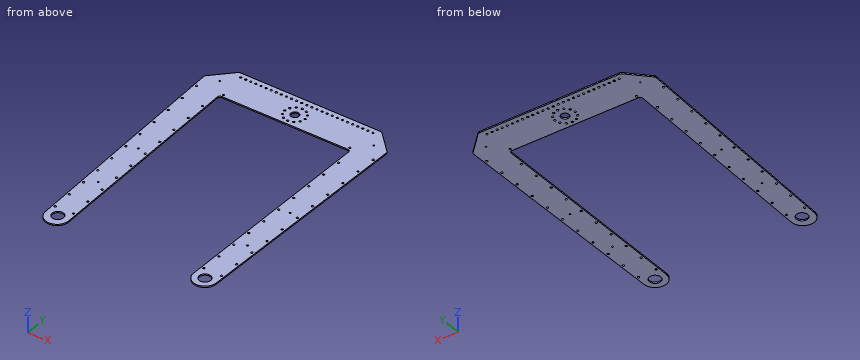
from build123d import *

# Parameters (mm, degrees)
SKETCH1_R           = 14.2875
SKETCH1_R_2         = 2.4892
SKETCH1_R_3         = 1.8288
SKETCH1_R_4         = 10.16
BOSS_EXTRUDE1_DEPTH = 3.175
FILLET1_R           = 6.35


with BuildPart() as part:
    # Sketch1 → Boss-Extrude1 (new body)
    with BuildSketch(Plane.XY):
        with BuildLine():
            Line((431.8, 25.4), (76.2, 25.4))
            Line((76.2, 25.4), (26.059319149, -25.4))
            Line((26.059319149, -25.4), (40.894, -596.9))
            ThreePointArc((40.894, -596.9), (69.687933371, -625.474161286), (98.040645192, -596.462146109))
            Line((98.040645192, -596.462146109), (89.873122894, -63.5))
            Line((89.873122894, -63.5), (418.126877106, -63.5))
            Line((418.126877106, -63.5), (409.959354808, -596.462146109))
            ThreePointArc((409.959354808, -596.462146109), (438.312066629, -625.474161286), (467.106, -596.9))
            Line((467.106, -596.9), (481.940680851, -25.4))
            Line((481.940680851, -25.4), (431.8, 25.4))
        make_face()
        with Locations((69.402383578, -593.962825081)):
            Circle(SKETCH1_R, mode=Mode.SUBTRACT)
        with Locations((46.582379595, -571.328944019)):
            Circle(SKETCH1_R_2, mode=Mode.SUBTRACT)
        with Locations((91.28656025, -570.142707564)):
            Circle(SKETCH1_R_2, mode=Mode.SUBTRACT)
        with Locations((45.264185314, -520.546049618)):
            Circle(SKETCH1_R_2, mode=Mode.SUBTRACT)
        with Locations((43.945991034, -469.763155216)):
            Circle(SKETCH1_R_2, mode=Mode.SUBTRACT)
        with Locations((90.508153333, -519.348671668)):
            Circle(SKETCH1_R_2, mode=Mode.SUBTRACT)
        with Locations((89.729746417, -468.554635771)):
            Circle(SKETCH1_R_2, mode=Mode.SUBTRACT)
        with Locations((67.240460084, -451.479225721)):
            Circle(SKETCH1_R_3, mode=Mode.SUBTRACT)
        with Locations((42.627796754, -418.980260814)):
            Circle(SKETCH1_R_2, mode=Mode.SUBTRACT)
        with Locations((88.9513395, -417.760599874)):
            Circle(SKETCH1_R_2, mode=Mode.SUBTRACT)
        with Locations((41.309602474, -368.197366412)):
            Circle(SKETCH1_R_2, mode=Mode.SUBTRACT)
        with Locations((39.991408193, -317.41447201)):
            Circle(SKETCH1_R_2, mode=Mode.SUBTRACT)
        with Locations((65.373280571, -308.991459085)):
            Circle(SKETCH1_R_3, mode=Mode.SUBTRACT)
        with Locations((88.172932583, -366.966563978)):
            Circle(SKETCH1_R_2, mode=Mode.SUBTRACT)
        with Locations((87.394525667, -316.172528081)):
            Circle(SKETCH1_R_2, mode=Mode.SUBTRACT)
        with Locations((416.71343975, -570.142707564)):
            Circle(SKETCH1_R_2, mode=Mode.SUBTRACT)
        with Locations((438.531, -596.9)):
            Circle(SKETCH1_R, mode=Mode.SUBTRACT)
        with Locations((461.417620405, -571.328944019)):
            Circle(SKETCH1_R_2, mode=Mode.SUBTRACT)
        with Locations((417.491846667, -519.348671668)):
            Circle(SKETCH1_R_2, mode=Mode.SUBTRACT)
        with Locations((418.270253583, -468.554635771)):
            Circle(SKETCH1_R_2, mode=Mode.SUBTRACT)
        with Locations((462.735814686, -520.546049618)):
            Circle(SKETCH1_R_2, mode=Mode.SUBTRACT)
        with Locations((464.054008966, -469.763155216)):
            Circle(SKETCH1_R_2, mode=Mode.SUBTRACT)
        with Locations((419.0486605, -417.760599874)):
            Circle(SKETCH1_R_2, mode=Mode.SUBTRACT)
        with Locations((442.219071981, -454.447733872)):
            Circle(SKETCH1_R_3, mode=Mode.SUBTRACT)
        with Locations((465.372203246, -418.980260814)):
            Circle(SKETCH1_R_2, mode=Mode.SUBTRACT)
        with Locations((419.827067417, -366.966563978)):
            Circle(SKETCH1_R_2, mode=Mode.SUBTRACT)
        with Locations((420.605474333, -316.172528081)):
            Circle(SKETCH1_R_2, mode=Mode.SUBTRACT)
        with Locations((466.690397526, -368.197366412)):
            Circle(SKETCH1_R_2, mode=Mode.SUBTRACT)
        with Locations((445.916762629, -311.995717095)):
            Circle(SKETCH1_R_3, mode=Mode.SUBTRACT)
        with Locations((468.008591807, -317.41447201)):
            Circle(SKETCH1_R_2, mode=Mode.SUBTRACT)
        with Locations((38.673213913, -266.631577608)):
            Circle(SKETCH1_R_2, mode=Mode.SUBTRACT)
        with Locations((86.61611875, -265.378492184)):
            Circle(SKETCH1_R_2, mode=Mode.SUBTRACT)
        with Locations((37.355019633, -215.848683206)):
            Circle(SKETCH1_R_2, mode=Mode.SUBTRACT)
        with Locations((36.036825353, -165.065788804)):
            Circle(SKETCH1_R_2, mode=Mode.SUBTRACT)
        with Locations((85.837711834, -214.584456288)):
            Circle(SKETCH1_R_2, mode=Mode.SUBTRACT)
        with Locations((85.059304917, -163.790420391)):
            Circle(SKETCH1_R_2, mode=Mode.SUBTRACT)
        with Locations((34.718631073, -114.282894402)):
            Circle(SKETCH1_R_2, mode=Mode.SUBTRACT)
        with Locations((33.400436792, -63.5)):
            Circle(SKETCH1_R_2, mode=Mode.SUBTRACT)
        with Locations((84.280898001, -112.996384494)):
            Circle(SKETCH1_R_2, mode=Mode.SUBTRACT)
        with Locations((61.612453458, -21.996099229)):
            Circle(SKETCH1_R_3, mode=Mode.SUBTRACT)
        with Locations((88.9, 12.7)):
            Circle(SKETCH1_R_2, mode=Mode.SUBTRACT)
        with Locations((101.6, 12.7)):
            Circle(SKETCH1_R_2, mode=Mode.SUBTRACT)
        with Locations((114.3, 12.7)):
            Circle(SKETCH1_R_2, mode=Mode.SUBTRACT)
        with Locations((127, 12.7)):
            Circle(SKETCH1_R_2, mode=Mode.SUBTRACT)
        with Locations((139.7, 12.7)):
            Circle(SKETCH1_R_2, mode=Mode.SUBTRACT)
        with Locations((152.4, 12.7)):
            Circle(SKETCH1_R_2, mode=Mode.SUBTRACT)
        with Locations((165.1, 12.7)):
            Circle(SKETCH1_R_2, mode=Mode.SUBTRACT)
        with Locations((177.8, 12.7)):
            Circle(SKETCH1_R_2, mode=Mode.SUBTRACT)
        with Locations((190.5, 12.7)):
            Circle(SKETCH1_R_2, mode=Mode.SUBTRACT)
        with Locations((203.2, 12.7)):
            Circle(SKETCH1_R_2, mode=Mode.SUBTRACT)
        with Locations((215.9, 12.7)):
            Circle(SKETCH1_R_2, mode=Mode.SUBTRACT)
        with Locations((228.6, 12.7)):
            Circle(SKETCH1_R_2, mode=Mode.SUBTRACT)
        with Locations((241.3, 12.7)):
            Circle(SKETCH1_R_2, mode=Mode.SUBTRACT)
        with Locations((421.38388125, -265.378492184)):
            Circle(SKETCH1_R_2, mode=Mode.SUBTRACT)
        with Locations((469.326786087, -266.631577608)):
            Circle(SKETCH1_R_2, mode=Mode.SUBTRACT)
        with Locations((422.162288166, -214.584456288)):
            Circle(SKETCH1_R_2, mode=Mode.SUBTRACT)
        with Locations((422.940695083, -163.790420391)):
            Circle(SKETCH1_R_2, mode=Mode.SUBTRACT)
        with Locations((470.644980367, -215.848683206)):
            Circle(SKETCH1_R_2, mode=Mode.SUBTRACT)
        with Locations((471.963174647, -165.065788804)):
            Circle(SKETCH1_R_2, mode=Mode.SUBTRACT)
        with Locations((254, 12.7)):
            Circle(SKETCH1_R_2, mode=Mode.SUBTRACT)
        with Locations((266.7, 12.7)):
            Circle(SKETCH1_R_2, mode=Mode.SUBTRACT)
        with Locations((279.4, 12.7)):
            Circle(SKETCH1_R_2, mode=Mode.SUBTRACT)
        with Locations((292.1, 12.7)):
            Circle(SKETCH1_R_2, mode=Mode.SUBTRACT)
        with Locations((304.8, 12.7)):
            Circle(SKETCH1_R_2, mode=Mode.SUBTRACT)
        with Locations((317.5, 12.7)):
            Circle(SKETCH1_R_2, mode=Mode.SUBTRACT)
        with Locations((330.2, 12.7)):
            Circle(SKETCH1_R_2, mode=Mode.SUBTRACT)
        with Locations((342.9, 12.7)):
            Circle(SKETCH1_R_2, mode=Mode.SUBTRACT)
        with Locations((355.6, 12.7)):
            Circle(SKETCH1_R_2, mode=Mode.SUBTRACT)
        with Locations((423.719101999, -112.996384494)):
            Circle(SKETCH1_R_2, mode=Mode.SUBTRACT)
        with Locations((473.281368927, -114.282894402)):
            Circle(SKETCH1_R_2, mode=Mode.SUBTRACT)
        with Locations((474.599563208, -63.5)):
            Circle(SKETCH1_R_2, mode=Mode.SUBTRACT)
        with Locations((368.3, 12.7)):
            Circle(SKETCH1_R_2, mode=Mode.SUBTRACT)
        with Locations((381, 12.7)):
            Circle(SKETCH1_R_2, mode=Mode.SUBTRACT)
        with Locations((393.7, 12.7)):
            Circle(SKETCH1_R_2, mode=Mode.SUBTRACT)
        with Locations((406.4, 12.7)):
            Circle(SKETCH1_R_2, mode=Mode.SUBTRACT)
        with Locations((419.1, 12.7)):
            Circle(SKETCH1_R_2, mode=Mode.SUBTRACT)
        with Locations((446.387546542, -21.996099229)):
            Circle(SKETCH1_R_3, mode=Mode.SUBTRACT)
        with Locations((266.7, -6.577954744)):
            Circle(SKETCH1_R_2, mode=Mode.SUBTRACT)
        with Locations((254, -3.175)):
            Circle(SKETCH1_R_2, mode=Mode.SUBTRACT)
        with Locations((411.873443795, -57.15)):
            Circle(SKETCH1_R_2, mode=Mode.SUBTRACT)
        with Locations((96.126556205, -57.15)):
            Circle(SKETCH1_R_2, mode=Mode.SUBTRACT)
        with Locations((232.002954744, -41.275)):
            Circle(SKETCH1_R_2, mode=Mode.SUBTRACT)
        with Locations((241.3, -50.572045256)):
            Circle(SKETCH1_R_2, mode=Mode.SUBTRACT)
        with Locations((228.6, -28.575)):
            Circle(SKETCH1_R_2, mode=Mode.SUBTRACT)
        with Locations((232.002954744, -15.875)):
            Circle(SKETCH1_R_2, mode=Mode.SUBTRACT)
        with Locations((241.3, -6.577954744)):
            Circle(SKETCH1_R_2, mode=Mode.SUBTRACT)
        with Locations((254, -53.975)):
            Circle(SKETCH1_R_2, mode=Mode.SUBTRACT)
        with Locations((266.7, -50.572045256)):
            Circle(SKETCH1_R_2, mode=Mode.SUBTRACT)
        with Locations((275.997045256, -41.275)):
            Circle(SKETCH1_R_2, mode=Mode.SUBTRACT)
        with Locations((254, -28.575)):
            Circle(SKETCH1_R_4, mode=Mode.SUBTRACT)
        with Locations((279.4, -28.575)):
            Circle(SKETCH1_R_2, mode=Mode.SUBTRACT)
        with Locations((275.997045256, -15.875)):
            Circle(SKETCH1_R_2, mode=Mode.SUBTRACT)
    extrude(amount=BOSS_EXTRUDE1_DEPTH)

    # Fillet1
    fillet1_edges = [part.edges().sort_by_distance(p)[0] for p in [
        (26.059319149, -25.4, 1.5875),
        (76.2, 25.4, 1.5875),
        (431.8, 25.4, 1.5875),
        (481.940680851, -25.4, 1.5875),
        (418.126877106, -63.5, 1.5875),
        (89.873122894, -63.5, 1.5875),
    ]]
    fillet(fillet1_edges, radius=FILLET1_R)


solid = part.part
The listing builds one solid part. Answer for the finished solid, in the listing's coordinates (mm). Give positions to 0.01 mm unless a question says otherwise; leave off trailing zeros. Loops run counter-clockwise (first coordinate to the right, second up) from the corner with the lowest first, then second, coordinate; pieces in that order, holes last. Notation, with made-up numbers: (17, -25.5) - (44, -25.5) arc R19 cw to (44, 10.5) - close; hole circle Ø9 at (3.5, 11). An arc over 180 degrees is marked (long way). Answer as a JSON object with one key per item and string values.
1. A cutting plane is placed at A-A (y = -277). Write down the section's boundary in (x, z) (3 decimals), then the cut area to 3 significant figures.
Determined:
{"outline": "(32.59, 0) - (93.145, 0) - (93.145, 3.175) - (32.59, 3.175) - close; (414.855, 0) - (475.41, 0) - (475.41, 3.175) - (414.855, 3.175) - close", "area": "385 mm²"}
2. Find the intervals of material crossed by L1, parallel to Y at x = 388, z = 1.25; L2, parallel to X at y = -41.5, z = 2.5; L3, parallel to X at y = -415.5, z = 2.95, in increasing order. Write a range as [from, to].
Determined:
{"L1": "[-63.5, 25.4]", "L2": "[26.48, 229.52], [234.48, 273.52], [278.48, 481.52]", "L3": "[36.19, 87.91], [89.99, 95.27], [412.73, 418.01], [420.09, 471.81]"}
3. Flat-ended cylindrical pins translate along their axes: pin 1 Ø1.5 at (y, z) = (-305, 2.5) entering from -X; pin 2 Ø1 at (x, z) = (319, 1.5) entering from -Y. Find the tip coordinate at first contact, or state that the pin passes through.
Determined:
{"pin 1": "x = 33.3", "pin 2": "y = -63.5"}
4. A cutting plane is placed at B-B (y = -508.5). Write down the section's boundary in (x, z) (3 decimals).
Determined:
{"outline": "(38.599, 0) - (96.693, 0) - (96.693, 3.175) - (38.599, 3.175) - close; (411.307, 0) - (469.401, 0) - (469.401, 3.175) - (411.307, 3.175) - close"}
5. A cutting plane is placed at C-C (z = 2.5). Give the number of separate pieces and of enclosed holes in the cut face, then the cut area to 3 significant figures.
Determined:
{"separate pieces": "1", "enclosed holes": "92", "area": "101,000 mm²"}
